from build123d import *

# Parameters (mm, degrees)
SKETCH1_W           = 120.65
SKETCH1_H           = 119.0625
BOSS_EXTRUDE1_DEPTH = 7.62
BOSS_EXTRUDE1_TAPER = 4
FILLET1_R           = 5.08
FILLET2_R           = 0.254
SHELL1_T            = -1.778
SKETCH5_R           = 2.38125
CUT_EXTRUDE1_DEPTH  = 8.6200001
SKETCH6_R           = 15.13967
SKETCH6_R_2         = 8.128
CUT_EXTRUDE2_DEPTH  = 8.6200001


with BuildPart() as part:
    # Sketch1 → Boss-Extrude1 (new body)
    with BuildSketch(Plane.XY):
        Rectangle(SKETCH1_W, SKETCH1_H)
    extrude(amount=BOSS_EXTRUDE1_DEPTH, taper=BOSS_EXTRUDE1_TAPER)

    # Fillet1
    fillet1_edges = [part.edges().sort_by_distance(p)[0] for p in [
        (-60.058578385, 59.264828385, 3.810006606),
        (60.058578385, 59.264828385, 3.810006606),
        (60.058578385, -59.264828385, 3.810006606),
        (-60.058578846, -59.264828846, 3.81),
    ]]
    fillet(fillet1_edges, radius=FILLET1_R)

    # Fillet2
    fillet2_edges = [part.edges().sort_by_distance(p)[0] for p in [
        (0, -58.998407693, 7.62),
        (-59.792157693, 0, 7.62),
        (59.792157693, 0, 7.62),
        (0, 58.998407693, 7.62),
        (-58.30937708, 57.51562708, 7.62),
        (58.30937708, 57.51562708, 7.62),
        (58.30937708, -57.51562708, 7.62),
        (-58.30937708, -57.51562708, 7.62),
    ]]
    fillet(fillet2_edges, radius=FILLET2_R)

    # Shell1
    shell1_openings = [part.faces().sort_by_distance(p)[0] for p in [
        (0, 0, 0),
    ]]
    offset(amount=SHELL1_T, openings=shell1_openings, kind=Kind.INTERSECTION)

    # Sketch5 → Cut-Extrude1 (cut, through all)
    with BuildSketch(Plane.XY.offset(7.62)):
        with Locations((-23.01875, 42.037)):
            Circle(SKETCH5_R)
        with Locations((-23.01875, -42.037)):
            Circle(SKETCH5_R)
        with Locations((23.01875, -42.037)):
            Circle(SKETCH5_R)
        with Locations((23.01875, 42.037)):
            Circle(SKETCH5_R)
    extrude(amount=-CUT_EXTRUDE1_DEPTH, mode=Mode.SUBTRACT)

    # Sketch6 → Cut-Extrude2 (cut, through all)
    with BuildSketch(Plane.XY.offset(7.62)):
        with Locations((23.01875, 0)):
            Circle(SKETCH6_R)
        with Locations((-35.51555, 12.4968)):
            Circle(SKETCH6_R_2)
        with Locations((-10.52195, 12.4968)):
            Circle(SKETCH6_R_2)
        with Locations((-10.52195, -12.4968)):
            Circle(SKETCH6_R_2)
        with Locations((-35.51555, -12.4968)):
            Circle(SKETCH6_R_2)
    extrude(amount=-CUT_EXTRUDE2_DEPTH, mode=Mode.SUBTRACT)


solid = part.part
Geometry: final body of the model. Coordinates: model frame, mm. A direction names the side the tool comes from. Round coordinates to 2 decimals unless told otherwise and drop trailing zeros. Loops run counter-clockwise (first coordinate to the right, second up) from the corner with the lowest first, then second, coordinate; pieces in that order, holes last.
Q1. Pull-direction query (Y, two-part tool) for faces 1 (the cylindrical face through (-6.771, 5.286, 6.743)), 2 (the cylindrical face through (-58.62, -57.74, 3.79)), 3 (the cylindrical face through (-58.62, 57.74, 3.79)); classes: released by +Y, released by -Y, zero draft, split by the parting line, or undercut.
Q2. Pin query (flat end, axial travel): P1, Ø1, axis at y = 31, z = 4, coming from the +X side; P2, Ø18.5, axis at x = -10.52, y = -12.5, coming from the -Z side; P3, Ø3, axis at x = -9.5, z = 2, coming from the -Y side. Return the tip coordinate at first contact, or that it passes through.
Q3. Material intervals for L1, parallel to Y at x = -22, z = 7; L2, parallel to Y at x = -46, z = 7.25; L3, parallel to Y at x = -53, z = 2.25, sorted ascending.
Q4. Access query for faces 4 (the flat face through (0.774, -59.277, 3.64)), 5 (the flat face through (58.34, 0.76, 2.88)). Directions: +Z, -Z, +X, -X, +Y, -Y. A direction counts if a zero-diameter tool reaches every point of the face in a straight line with its end or side. Return the directions, or none.
Q5. Section A-A on y = 0. Return loops of the section in (x, z) (3 decimals), plus the area to 3 significant figures.
Q6. Section B-B on x = 3.5. Return loops of the section in (y, z), plus the area to 3 significant figures.
Q7. Section C-C on y = -17. Return loops of the section in (x, z) (3 decimals), plus the area to 3 significant figures.
Evaluation:
1. face 1: undercut
1. face 2: released by -Y
1. face 3: released by +Y
2. P1: stops at x = 60.08
2. P2: stops at z = 5.84
2. P3: stops at y = -59.5
3. L1: y = -59.04 to -44.19, -39.88 to 39.88, 44.19 to 59.04
3. L2: y = -59.02 to 59.02
3. L3: y = -59.37 to -57.59, 57.59 to 59.37
4. face 4: +Z, +X, -X, -Y
4. face 5: -Z
5. outline: (-60.325, 0) - (-58.543, 0) - (-58.134, 5.842) - (7.879, 5.842) - (7.879, 7.62) - (-59.555, 7.62) arc R0.254 ccw to (-59.809, 7.384) - close; (38.158, 5.842) - (58.134, 5.842) - (58.543, 0) - (60.325, 0) - (59.809, 7.384) arc R0.254 ccw to (59.555, 7.62) - (38.158, 7.62) - close
5. area: 180 mm2
6. outline: (-59.53, 0) - (-57.75, 0) - (-57.34, 5.84) - (57.34, 5.84) - (57.75, 0) - (59.53, 0) - (59.01, 7.38) arc R0.25 ccw to (58.76, 7.62) - (-58.76, 7.62) arc R0.25 ccw to (-59.01, 7.38) - close
6. area: 231 mm2
7. outline: (-60.325, 0) - (-58.543, 0) - (-58.134, 5.842) - (-42.282, 5.842) - (-42.282, 7.62) - (-59.555, 7.62) arc R0.254 ccw to (-59.809, 7.384) - close; (-28.749, 5.842) - (-17.288, 5.842) - (-17.288, 7.62) - (-28.749, 7.62) - close; (-3.755, 5.842) - (58.134, 5.842) - (58.543, 0) - (60.325, 0) - (59.809, 7.384) arc R0.254 ccw to (59.555, 7.62) - (-3.755, 7.62) - close
7. area: 186 mm2
